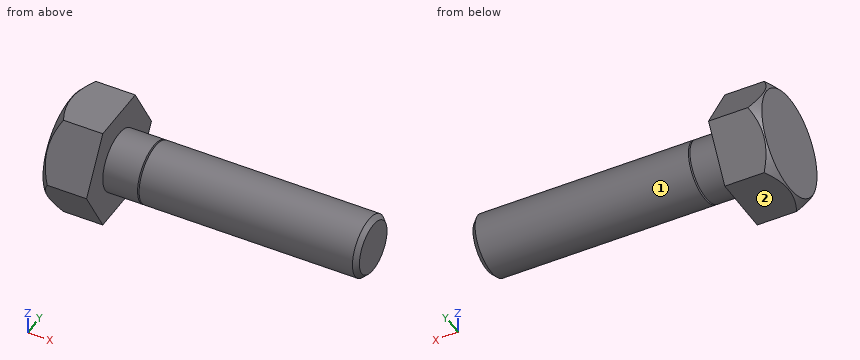
```python
from build123d import *

# Parameters (mm, degrees)
F2_SIZE  = 1.5
F4_DEPTH = 50.001


with BuildPart() as f1:
    # F0 (on Front) → F1 (revolve)
    with BuildSketch(Plane.XZ):
        Polygon((8, 5), (8, 10), (0, 10), (0, 0), (50, 0), (50, 4.25), (49.25, 5), (14, 5), (13.875, 4.25), (13.75, 5), align=None)
    revolve(axis=Axis((25, 0, 0), (1, 0, 0)))

    # F2
    f2_edges = [f1.edges().sort_by_distance(p)[0] for p in [
        (0, 0, -10),
    ]]
    chamfer(f2_edges, length=F2_SIZE)

    # F3 (on face) → F4 (cut, through all)
    with BuildSketch(Plane(origin=(0, 0, 0), x_dir=(0, -1, 0), z_dir=(-1, 0, 0))):
        with BuildLine():
            Line((-10, 0), (-5, 8.660254))
            ThreePointArc((-5, 8.660254), (-8.660254, 5), (-10, 0))
        make_face()
        with BuildLine():
            Line((-5, 8.660254), (5, 8.660254))
            ThreePointArc((5, 8.660254), (0, 10), (-5, 8.660254))
        make_face()
        with BuildLine():
            Line((5, 8.660254), (10, 0))
            ThreePointArc((10, 0), (8.660254, 5), (5, 8.660254))
        make_face()
        with BuildLine():
            ThreePointArc((5, -8.660254), (8.660254, -5), (10, 0))
            Line((10, 0), (5, -8.660254))
        make_face()
        with BuildLine():
            ThreePointArc((-5, -8.660254), (0, -10), (5, -8.660254))
            Line((5, -8.660254), (-5, -8.660254))
        make_face()
        with BuildLine():
            ThreePointArc((-10, 0), (-8.660254, -5), (-5, -8.660254))
            Line((-5, -8.660254), (-10, 0))
        make_face()
    extrude(amount=-F4_DEPTH, mode=Mode.SUBTRACT)


solid = f1.part
```
Geometry: final body of the model. Coordinates: model frame, mm. Face numbers are marked on the shaded views. A direction names the side the tool comes from. Round coordinates to 2 decimals unless told otherwise and drop trailing zeros. Order: outer loops, then holes, each group sorted by start corner. A loop starts at its lowest first (then second) coordinate and runs counter-clockwise, first axis right, second up. Notation, with made-up numbers: (11, -7) -> (31, -7) arc R34 ccw to (31, 24) -> close; hole circle Ø5 at (18, 64.25). An arc over 180 degrees is marked (long way). Use CSV: the item, a comma, the result in double quotes. Start each with the question number.
1) Material intervals for line 1 along X through (y, z) = (0.25, -5.5); line 2 along Z through (x, y) = (46.5, 1.5); line 3 along Y through (x, z) = (33, -2.5), sorted ascending. Write a range as from..to.
2) Set-up query: the marked faces 1 and 2. Return all of +Z, -Z, +X, -X, +Y, -Y with unobstructed straight access to the full face (end or side cutting, diameter ignored); none if empty.
3) Section B-B (x = 26.5). Return the cut outline in (y, z).
4) First-contact query: pin 1 Ø1 at (x, z) = (34, 3.5) entering from -Y; pin 2 Ø5 at (x, z) = (32.5, 1.5) entering from +Y; pin 3 Ø1 at (x, y) = (28.5, 1.5) entering from -Z. Flat tips, straight axial feed; report the tip coordinate or a pass-through.
5) Section A-A (y = 0). Return the cut outline in (x, z) (3 decimals), and give its area (3 significant figures).
Returned:
1,line 1,"x = 0..8"
1,line 2,"z = -4.77..4.77"
1,line 3,"y = -4.33..4.33"
2,face 1,"+X"
2,face 2,"-Z, +X, -X, +Y, -Y"
3,outline,"circle Ø10 at (0, 0)"
4,pin 1,"stops at y = -4"
4,pin 2,"stops at y = 5"
4,pin 3,"stops at z = -4.9"
5,outline,"(0, -8.5) -> (0.16, -8.66) -> (8, -8.66) -> (8, -5) -> (13.75, -5) -> (13.875, -4.25) -> (14, -5) -> (49.25, -5) -> (50, -4.25) -> (50, 4.25) -> (49.25, 5) -> (14, 5) -> (13.875, 4.25) -> (13.75, 5) -> (8, 5) -> (8, 8.66) -> (0.16, 8.66) -> (0, 8.5) -> close"
5,area,"558 mm²"
